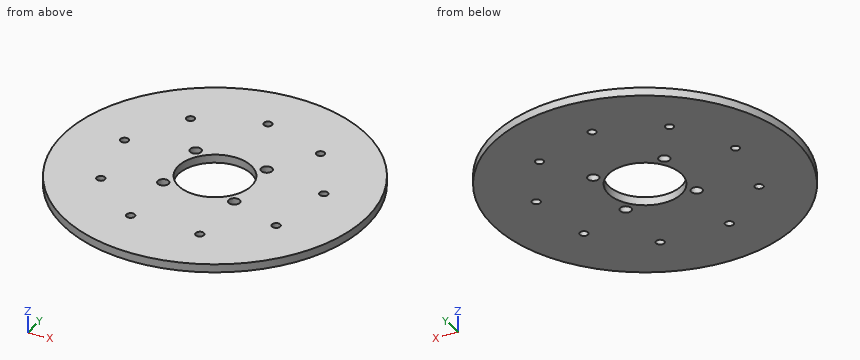
from build123d import *

# Parameters (mm, degrees)
SKETCH_1_R      = 55
SKETCH_1_R_2    = 1.5
SKETCH_1_R_3    = 13.25
SKETCH_1_R_4    = 2
EXTRUDE_1_DEPTH = 3


with BuildPart() as part:
    # 草图1 → 凸台-拉伸1 (new body)
    with BuildSketch(Plane.XY):
        Circle(SKETCH_1_R)
        with Locations((0, 36.5)):
            Circle(SKETCH_1_R_2, mode=Mode.SUBTRACT)
        with Locations((23.461747754, 27.960622174)):
            Circle(SKETCH_1_R_2, mode=Mode.SUBTRACT)
        with Locations((35.945482985, 6.338158485)):
            Circle(SKETCH_1_R_2, mode=Mode.SUBTRACT)
        with Locations((31.609927238, -18.25)):
            Circle(SKETCH_1_R_2, mode=Mode.SUBTRACT)
        with Locations((12.483735231, -34.298780659)):
            Circle(SKETCH_1_R_2, mode=Mode.SUBTRACT)
        with Locations((-12.483735231, -34.298780659)):
            Circle(SKETCH_1_R_2, mode=Mode.SUBTRACT)
        with Locations((-31.609927238, -18.25)):
            Circle(SKETCH_1_R_2, mode=Mode.SUBTRACT)
        with Locations((-35.945482985, 6.338158485)):
            Circle(SKETCH_1_R_2, mode=Mode.SUBTRACT)
        with Locations((-23.461747754, 27.960622174)):
            Circle(SKETCH_1_R_2, mode=Mode.SUBTRACT)
        Circle(SKETCH_1_R_3, mode=Mode.SUBTRACT)
        with Locations((-12.809350268, 11.176786018)):
            Circle(SKETCH_1_R_4, mode=Mode.SUBTRACT)
        with Locations(Location((12.809350268, 11.176786018, 0), (0, 0, 180))):
            Circle(SKETCH_1_R_4, mode=Mode.SUBTRACT)
        with Locations((12.809350268, -11.176786018)):
            Circle(SKETCH_1_R_4, mode=Mode.SUBTRACT)
        with Locations(Location((-12.809350268, -11.176786018, 0), (0, 0, 180))):
            Circle(SKETCH_1_R_4, mode=Mode.SUBTRACT)
    extrude(amount=EXTRUDE_1_DEPTH)


solid = part.part
Here's how the part is built. I have some questions about the finished solid (model axes, mm). Give positions to 0.01 mm unless a question says otherwise; leave off trailing zeros. Order: outer loops, then holes, each group sorted by start corner. A loop starts at its lowest first (then second) coordinate and runs counter-clockwise, first axis right, second up. Notation, with made-up numbers: (5, 45) -> (15, 45) arc R19 cw to (15, 70) -> close; hole circle Ø6 at (59, -7.5). An arc over 180 degrees is marked (long way). One line per item, written item: value. Start each with the question number.
1. Imagine slicing it at D-D, the plane z = 2.5. Count the separate pieces of the cut face and the enclosed holes in it, plus the area to 3 significant figures.
2. Will these pins go through, and if not, where does the flat tip stop? pin 1 Ø1 at (x, z) = (-31.5, 1) entering from +Y; pin 2 Ø1 at (x, z) = (4, 0.5) entering from -Y.
3. Imagine slicing it at B-B, the plane x = 0. List the corners of the cut face in (y, z) for me, plus the area to 4 significant figures.
4. Imagine slicing it at A-A, the plane y = 0. List the corners of the cut face in (x, z) for me, plus the area to 4 significant figures.
5. I need wall thicknesses on probe 1 along Y at (x, z) = (0, 2.55); probe 2 along X at (y, z) = (6, 1.7); probe 3 along X at (y, z) = (-10.5, 0.65). Which ranges of each line are inside material? Lowest first, please. Write a range as from..to.
6. Imagine slicing it at C-C, the plane y = -18.25. List the corners of the cut face in (x, z) for me.
Values follow:
1. separate pieces: 1
1. enclosed holes: 14
1. area: 8,840 mm2
2. pin 1: stops at y = 45.43
2. pin 2: stops at y = -54.89
3. outline: (-55, 0) -> (-13.25, 0) -> (-13.25, 3) -> (-55, 3) -> close; (13.25, 0) -> (35, 0) -> (35, 3) -> (13.25, 3) -> close; (38, 0) -> (55, 0) -> (55, 3) -> (38, 3) -> close
3. area: 241.5 mm2
4. outline: (-55, 0) -> (-13.25, 0) -> (-13.25, 3) -> (-55, 3) -> close; (13.25, 0) -> (55, 0) -> (55, 3) -> (13.25, 3) -> close
4. area: 250.5 mm2
5. probe 1: y = -55..-13.25, 13.25..35, 38..55
5. probe 2: x = -54.67..-37.41, -34.48..-11.81, 11.81..34.48, 37.41..54.67
5. probe 3: x = -53.99..-14.69, -10.93..-8.08, 8.08..10.93, 14.69..53.99
6. outline: (-51.88, 0) -> (-33.11, 0) -> (-33.11, 3) -> (-51.88, 3) -> close; (-30.11, 0) -> (30.11, 0) -> (30.11, 3) -> (-30.11, 3) -> close; (33.11, 0) -> (51.88, 0) -> (51.88, 3) -> (33.11, 3) -> close
